Input: part model. Units: mm. Frame: model coordinates. A direction names the side the tool comes from. Round coordinates to 2 decimals unless told otherwise and drop trailing zeros. Loops run counter-clockwise (first coordinate to the right, second up) from the corner with the lowest first, then second, coordinate; pieces in that order, holes last.
(1) Cut plane B-B, the plane x = 0. Output: boundary loops of the cut face in (y, z), and give its area (3 significant figures).
(2) Cut plane C-C, the plane x = 3.5. Output: boundary loops of the cut face in (y, z).
(3) Line query: line 1 (X direction, y = -11.5, z = 3.75); line 2 (X direction, y = -12, z = 6.75); line 3 (Y direction, x = 0, z = 4.25). Output: solid intervals per line, ascending.
(4) Draft query along Y for faces 6 (the face through (5.8, 13.61, 4.93)), 7 (the face through (-11.5, 4.9, 4.9)), 8 (the face through (3.67, -16.6, 4.93)). Return one class per face: released by +Y, released by -Y, zero draft, split by the parting line, or undercut.
(5) Cut plane A-A, the plane y = -2. Output: boundary loops of the cut face in (x, z).
(6) First-contact query: pin 1 Ø2 at (y, z) = (6.5, 3) entering from -X; pin 2 Ø1.5 at (y, z) = (7, 2) entering from +X. Flat tips, straight axial feed; report the tip coordinate or a pass-through.
(7) Access query for faces 1 (the face through (1.253, 14.673, 4.93)), 2 (the face through (-12.46, -1.02, 4.93)), 3 (the face through (-16.102, -5.451, 4.93)), 4 (the face through (14.1, 9.5, 4.9)), 5 (the face through (-5.11, -13.81, 4.93)). Directions: +Z, -Z, +X, -X, +Y, -Y. A direction counts if a zero-diameter tool reaches every point of the face in a straight line with its end or side. Return the directions, or none.
from build123d import *

# Parameters (mm, degrees)
F0_R     = 3.1
F1_DEPTH = 10


# Not quite as in the source:
# - a feature names something its author has since deleted; it is built from what else it names


with BuildPart() as f1:
    # F0 (on Top) → F1 (new body)
    with BuildSketch(Plane.XY):
        with BuildLine():
            Line((11.7831534795, -12.2946042669), (9.1877297548, -8.4755897702))
            ThreePointArc((9.1877297548, -8.4755897702), (8.1042674519, -9.516871811), (6.9036805201, -10.4206139587))
            Line((6.9036805201, -10.4206139587), (10.2604539897, -13.5912870592))
            Line((10.2604539897, -13.5912870592), (11.7831534795, -12.2946042669))
        make_face()
        with BuildLine():
            ThreePointArc((9.4254531567, 8.2104100258), (10.3425930143, 7.0200263348), (11.110259477, 5.7281877024))
            Line((11.110259477, 5.7281877024), (14.6275286062, 8.7198283742))
            Line((14.6275286062, 8.7198283742), (13.5043243926, 10.3746432565))
            Line((13.5043243926, 10.3746432565), (9.4254531567, 8.2104100258))
        make_face()
        with BuildLine():
            Line((16.1681140592, -5.3471569801), (12.0867087003, -3.1877065099))
            ThreePointArc((12.0867087003, -3.1877065099), (11.6168440528, -4.6150768414), (10.9790902584, -5.9757490826))
            Line((10.9790902584, -5.9757490826), (15.4297017645, -7.2058520285))
            Line((15.4297017645, -7.2058520285), (16.1681140592, -5.3471569801))
        make_face()
        with BuildLine():
            ThreePointArc((-6.6040163856, 10.6130564673), (-5.2827282718, 11.328847338), (-3.8850930245, 11.8809112526))
            Line((-3.8850930245, 11.8809112526), (-6.2782026626, 15.8298506414))
            Line((-6.2782026626, 15.8298506414), (-8.0908182366, 14.9846141179))
            Line((-8.0908182366, 14.9846141179), (-6.6040163856, 10.6130564673))
        make_face()
        with BuildLine():
            Line((-10.9387342022, -13.0515935446), (-7.4249743059, -10.0558319674))
            ThreePointArc((-7.4249743059, -10.0558319674), (-8.5780204734, -9.0921705197), (-9.6070952306, -7.9971070538))
            Line((-9.6070952306, -7.9971070538), (-12.3934814853, -11.6791102689))
            Line((-12.3934814853, -11.6791102689), (-10.9387342022, -13.0515935446))
        make_face()
        with BuildLine():
            ThreePointArc((4.484602064, 11.6678337461), (5.8523358933, 11.0453684679), (7.1354904963, 10.2632731318))
            Line((7.1354904963, 10.2632731318), (8.8428062923, 14.5535142449))
            Line((8.8428062923, 14.5535142449), (7.0755473374, 15.4898879879))
            Line((7.0755473374, 15.4898879879), (4.484602064, 11.6678337461))
        make_face()
        with BuildLine():
            ThreePointArc((-10.8043972519, 6.2860957696), (-9.9719920146, 7.5371994308), (-8.9954693884, 8.6793738531))
            Line((-8.9954693884, 8.6793738531), (-12.9589331854, 11.0483505871))
            Line((-12.9589331854, 11.0483505871), (-14.1648850944, 9.4528318648))
            Line((-14.1648850944, 9.4528318648), (-10.8043972519, 6.2860957696))
        make_face()
        with BuildLine():
            Line((-3.5552032377, -16.6541445274), (-1.8529176571, -12.3619050375))
            ThreePointArc((-1.8529176571, -12.3619050375), (-3.3229568779, -12.0502264538), (-4.744972006, -11.5643953868))
            Line((-4.744972006, -11.5643953868), (-5.4832394703, -16.1224714269))
            Line((-5.4832394703, -16.1224714269), (-3.5552032377, -16.6541445274))
        make_face()
        with BuildLine():
            ThreePointArc((-12.4901514097, 0.4961025726), (-12.340363914, 1.9913358508), (-12.0122308055, 3.457789912))
            Line((-12.0122308055, 3.457789912), (-16.6235880549, 3.6954458703))
            Line((-16.6235880549, 3.6954458703), (-16.9422017911, 1.720987644))
            Line((-16.9422017911, 1.720987644), (-12.4901514097, 0.4961025726))
        make_face()
        with BuildLine():
            Line((-15.7763727361, -6.4114010396), (-11.2689346746, -5.4093540556))
            ThreePointArc((-11.2689346746, -5.4093540556), (-11.8366266187, -4.0179933163), (-12.2332530705, -2.5685636671))
            Line((-12.2332530705, -2.5685636671), (-16.4192516667, -4.5175407807))
            Line((-16.4192516667, -4.5175407807), (-15.7763727361, -6.4114010396))
        make_face()
        with BuildLine():
            ThreePointArc((12.1726144308, 2.8420868951), (12.4178838854, 1.4304404243), (12.5, 0))
            ThreePointArc((12.5, 0), (12.4998037623, -0.0700421594), (12.4992150553, -0.1400821196))
            Line((12.4992150553, -0.1400821196), (17.0078246246, 0.8566805343))
            Line((17.0078246246, 0.8566805343), (16.7900908749, 2.8447932107))
            Line((16.7900908749, 2.8447932107), (12.1726144308, 2.8420868951))
        make_face()
        with BuildLine():
            Line((4.6557694441, -16.3805925071), (4.1503889837, -11.7908554093))
            ThreePointArc((4.1503889837, -11.7908554093), (2.7054951742, -12.203700089), (1.2215009624, -12.4401742511))
            Line((1.2215009624, -12.4401742511), (2.7031774298, -16.813471735))
            Line((2.7031774298, -16.813471735), (4.6557694441, -16.3805925071))
        make_face()
        with BuildLine():
            ThreePointArc((-1.5, 12.409673646), (0, 12.5), (1.5, 12.409673646))
            Line((1.5, 12.409673646), (1, 17))
            Line((1, 17), (-1, 17))
            Line((-1, 17), (-1.5, 12.409673646))
        make_face()
        with BuildLine():
            ThreePointArc((-4.744972006, -11.5643953868), (-3.3229568779, -12.0502264538), (-1.8529176571, -12.3619050375))
            Line((-1.8529176571, -12.3619050375), (-4.744972006, -11.5643953868))
        make_face()
        with BuildLine():
            Line((4.484602064, 11.6678337461), (7.1354904963, 10.2632731318))
            ThreePointArc((7.1354904963, 10.2632731318), (5.8523358933, 11.0453684679), (4.484602064, 11.6678337461))
        make_face()
        with BuildLine():
            Line((-10.8043972519, 6.2860957696), (-8.9954693884, 8.6793738531))
            ThreePointArc((-8.9954693884, 8.6793738531), (-9.9719920146, 7.5371994308), (-10.8043972519, 6.2860957696))
        make_face()
        with BuildLine():
            ThreePointArc((-12.2332530705, -2.5685636671), (-11.8366266187, -4.0179933163), (-11.2689346746, -5.4093540556))
            Line((-11.2689346746, -5.4093540556), (-12.2332530705, -2.5685636671))
        make_face()
        with BuildLine():
            ThreePointArc((10.9790902584, -5.9757490826), (11.6168440528, -4.6150768414), (12.0867087003, -3.1877065099))
            Line((12.0867087003, -3.1877065099), (10.9790902584, -5.9757490826))
        make_face()
        with BuildLine():
            Line((-12.4901514097, 0.4961025726), (-12.0122308055, 3.457789912))
            ThreePointArc((-12.0122308055, 3.457789912), (-12.340363914, 1.9913358508), (-12.4901514097, 0.4961025726))
        make_face()
        with BuildLine():
            ThreePointArc((-9.6070952306, -7.9971070538), (-8.5780204734, -9.0921705197), (-7.4249743059, -10.0558319674))
            Line((-7.4249743059, -10.0558319674), (-9.6070952306, -7.9971070538))
        make_face()
        with BuildLine():
            ThreePointArc((12.4992150553, -0.1400821196), (12.4998037623, -0.0700421594), (12.5, 0))
            ThreePointArc((12.5, 0), (12.4178838854, 1.4304404243), (12.1726144308, 2.8420868951))
            Line((12.1726144308, 2.8420868951), (12.4992150553, -0.1400821196))
        make_face()
        with BuildLine():
            Line((-6.6040163856, 10.6130564673), (-3.8850930245, 11.8809112526))
            ThreePointArc((-3.8850930245, 11.8809112526), (-5.2827282718, 11.328847338), (-6.6040163856, 10.6130564673))
        make_face()
        with BuildLine():
            ThreePointArc((1.2215009624, -12.4401742511), (2.7054951742, -12.203700089), (4.1503889837, -11.7908554093))
            Line((4.1503889837, -11.7908554093), (1.2215009624, -12.4401742511))
        make_face()
        with BuildLine():
            Line((9.4254531567, 8.2104100258), (11.110259477, 5.7281877024))
            ThreePointArc((11.110259477, 5.7281877024), (10.3425930143, 7.0200263348), (9.4254531567, 8.2104100258))
        make_face()
        with BuildLine():
            ThreePointArc((6.9036805201, -10.4206139587), (8.1042674519, -9.516871811), (9.1877297548, -8.4755897702))
            Line((9.1877297548, -8.4755897702), (6.9036805201, -10.4206139587))
        make_face()
        with BuildLine():
            Line((-1.5, 12.409673646), (1.5, 12.409673646))
            ThreePointArc((1.5, 12.409673646), (0, 12.5), (-1.5, 12.409673646))
        make_face()
        with BuildLine():
            Line((12.4992150553, -0.1400821196), (12.1726144308, 2.8420868951))
            ThreePointArc((12.1726144308, 2.8420868951), (11.7305348906, 4.3179336703), (11.110259477, 5.7281877024))
            Line((11.110259477, 5.7281877024), (9.4254531567, 8.2104100258))
            ThreePointArc((9.4254531567, 8.2104100258), (8.3438465591, 9.3075359037), (7.1354904963, 10.2632731318))
            Line((7.1354904963, 10.2632731318), (4.484602064, 11.6678337461))
            ThreePointArc((4.484602064, 11.6678337461), (3.0152026591, 12.1308925032), (1.5, 12.409673646))
            Line((1.5, 12.409673646), (-1.5, 12.409673646))
            ThreePointArc((-1.5, 12.409673646), (-2.7054951742, 12.203700089), (-3.8850930245, 11.8809112526))
            Line((-3.8850930245, 11.8809112526), (-6.6040163856, 10.6130564673))
            ThreePointArc((-6.6040163856, 10.6130564673), (-7.8594383525, 9.7200426328), (-8.9954693884, 8.6793738531))
            Line((-8.9954693884, 8.6793738531), (-10.8043972519, 6.2860957696))
            ThreePointArc((-10.8043972519, 6.2860957696), (-11.4956277551, 4.9092303386), (-12.0122308055, 3.457789912))
            Line((-12.0122308055, 3.457789912), (-12.4901514097, 0.4961025726))
            ThreePointArc((-12.4901514097, 0.4961025726), (-12.4563127395, -1.0441613555), (-12.2332530705, -2.5685636671))
            Line((-12.2332530705, -2.5685636671), (-11.2689346746, -5.4093540556))
            ThreePointArc((-11.2689346746, -5.4093540556), (-10.5179024784, -6.7545338443), (-9.6070952306, -7.9971070538))
            Line((-9.6070952306, -7.9971070538), (-7.4249743059, -10.0558319674))
            ThreePointArc((-7.4249743059, -10.0558319674), (-6.131544602, -10.8928490669), (-4.744972006, -11.5643953868))
            Line((-4.744972006, -11.5643953868), (-1.8529176571, -12.3619050375))
            ThreePointArc((-1.8529176571, -12.3619050375), (-0.3181246266, -12.4959512132), (1.2215009624, -12.4401742511))
            Line((1.2215009624, -12.4401742511), (4.1503889837, -11.7908554093))
            ThreePointArc((4.1503889837, -11.7908554093), (5.5693360069, -11.1907326142), (6.9036805201, -10.4206139587))
            Line((6.9036805201, -10.4206139587), (9.1877297548, -8.4755897702))
            ThreePointArc((9.1877297548, -8.4755897702), (10.1605835574, -7.2809712108), (10.9790902584, -5.9757490826))
            Line((10.9790902584, -5.9757490826), (12.0867087003, -3.1877065099))
            ThreePointArc((12.0867087003, -3.1877065099), (12.3870462717, -1.6766289583), (12.4992150553, -0.1400821196))
        make_face()
        Circle(F0_R, mode=Mode.SUBTRACT)
    extrude(amount=F1_DEPTH)


solid = f1.part
Reported:
1. outline: (-12.5, 0) - (-3.1, 0) - (-3.1, 10) - (-12.5, 10) - close; (3.1, 0) - (17, 0) - (17, 10) - (3.1, 10) - close
1. area: 233 mm2
2. outline: (-16.64, 0) - (12, 0) - (12, 10) - (-16.64, 10) - close
3. line 1: x = -12.26 to -9.12, -4.9 to 4.9, 8.05 to 11.24
3. line 2: x = -12.05 to -9.71, -4.82 to 4.17, 8.58 to 11.58
3. line 3: y = -12.5 to -3.1, 3.1 to 17
4. face 6: released by +Y
4. face 7: undercut
4. face 8: released by -Y
5. outline: (-12.34, 0) - (-2.37, 0) - (-2.37, 10) - (-12.34, 10) - close; (2.37, 0) - (12.34, 0) - (12.34, 10) - (2.37, 10) - close
6. pin 1: stops at x = -12.09
6. pin 2: stops at x = 13.49
7. face 1: +Z, -Z, +Y
7. face 2: +Z, -Z, -X
7. face 3: +Z, -Z, -X, -Y
7. face 4: +Z, -Z, +X, +Y
7. face 5: +Z, -Z
